```python
from build123d import *

# Parameters (mm, degrees)
F0_R     = 4.5
F1_DEPTH = 10


with BuildPart() as f1:
    # F0 (on Top) → F1 (new body)
    with BuildSketch(Plane.XY):
        with BuildLine():
            ThreePointArc((-2.392851, 5.821348), (-2.36707, 5.442285), (-2.615174, 5.154538))
            ThreePointArc((-2.615174, 5.154538), (-2.753594, 5.081941), (-2.89, 5.005627))
            ThreePointArc((-2.89, 5.005627), (-3.024293, 4.925652), (-3.156374, 4.842076))
            ThreePointArc((-3.156374, 4.842076), (-3.529622, 4.771085), (-3.84501, 4.982943))
            ThreePointArc((-3.84501, 4.982943), (-5.394961, 6.242549), (-7.385022, 6.411696))
            Line((-7.385022, 6.411696), (-7.492977, 6.287354))
            Line((-7.492977, 6.287354), (-7.596684, 6.159448))
            ThreePointArc((-7.596684, 6.159448), (-7.084536, 4.228992), (-5.57492, 2.921316))
            ThreePointArc((-5.57492, 2.921316), (-5.311514, 2.647509), (-5.316613, 2.267604))
            ThreePointArc((-5.316613, 2.267604), (-5.375984, 2.123017), (-5.431423, 1.976876))
            ThreePointArc((-5.431423, 1.976876), (-5.482891, 1.829291), (-5.53035, 1.680367))
            ThreePointArc((-5.53035, 1.680367), (-5.770641, 1.386066), (-6.148423, 1.345631))
            ThreePointArc((-6.148423, 1.345631), (-8.145413, 1.314256), (-9.778614, 0.164643))
            Line((-9.778614, 0.164643), (-9.781386, 0))
            Line((-9.781386, 0), (-9.778614, -0.164643))
            ThreePointArc((-9.778614, -0.164643), (-8.145413, -1.314256), (-6.148423, -1.345631))
            ThreePointArc((-6.148423, -1.345631), (-5.770641, -1.386066), (-5.53035, -1.680367))
            ThreePointArc((-5.53035, -1.680367), (-5.482891, -1.829291), (-5.431423, -1.976876))
            ThreePointArc((-5.431423, -1.976876), (-5.375984, -2.123017), (-5.316613, -2.267604))
            ThreePointArc((-5.316613, -2.267604), (-5.311514, -2.647509), (-5.57492, -2.921316))
            ThreePointArc((-5.57492, -2.921316), (-7.084536, -4.228992), (-7.596684, -6.159448))
            Line((-7.596684, -6.159448), (-7.492977, -6.287354))
            Line((-7.492977, -6.287354), (-7.385022, -6.411696))
            ThreePointArc((-7.385022, -6.411696), (-5.394961, -6.242549), (-3.84501, -4.982943))
            ThreePointArc((-3.84501, -4.982943), (-3.529622, -4.771085), (-3.156374, -4.842076))
            ThreePointArc((-3.156374, -4.842076), (-3.024293, -4.925652), (-2.89, -5.005627))
            ThreePointArc((-2.89, -5.005627), (-2.753594, -5.081941), (-2.615174, -5.154538))
            ThreePointArc((-2.615174, -5.154538), (-2.36707, -5.442285), (-2.392851, -5.821348))
            ThreePointArc((-2.392851, -5.821348), (-2.708726, -7.793448), (-1.860181, -9.601465))
            Line((-1.860181, -9.601465), (-1.69852, -9.632785))
            Line((-1.69852, -9.632785), (-1.535897, -9.658645))
            ThreePointArc((-1.535897, -9.658645), (-0.120147, -8.249884), (0.257526, -6.288681))
            ThreePointArc((0.257526, -6.288681), (0.362947, -5.92366), (0.694504, -5.738124))
            ThreePointArc((0.694504, -5.738124), (0.849406, -5.717247), (1.003686, -5.692189))
            ThreePointArc((1.003686, -5.692189), (1.157233, -5.662968), (1.309934, -5.629607))
            ThreePointArc((1.309934, -5.629607), (1.684953, -5.690555), (1.90886, -5.997506))
            ThreePointArc((1.90886, -5.997506), (2.934527, -7.711263), (4.746722, -8.55085))
            Line((4.746722, -8.55085), (4.890693, -8.470929))
            Line((4.890693, -8.470929), (5.031892, -8.386207))
            ThreePointArc((5.031892, -8.386207), (5.210886, -6.397007), (4.239562, -4.651875))
            ThreePointArc((4.239562, -4.651875), (4.085689, -4.304489), (4.220415, -3.94924))
            ThreePointArc((4.220415, -3.94924), (4.325658, -3.833678), (4.427737, -3.715312))
            ThreePointArc((4.427737, -3.715312), (4.526578, -3.59423), (4.622109, -3.47052))
            ThreePointArc((4.622109, -3.47052), (4.948567, -3.276151), (5.317394, -3.367364))
            ThreePointArc((5.317394, -3.367364), (7.204682, -4.020892), (9.13258, -3.499197))
            Line((9.13258, -3.499197), (9.191496, -3.345431))
            Line((9.191496, -3.345431), (9.245203, -3.189769))
            ThreePointArc((9.245203, -3.189769), (8.103686, -1.550899), (6.23786, -0.838405))
            ThreePointArc((6.23786, -0.838405), (5.896692, -0.6712), (5.771548, -0.312462))
            ThreePointArc((5.771548, -0.312462), (5.777887, -0.156288), (5.78, 0))
            ThreePointArc((5.78, 0), (5.777887, 0.156288), (5.771548, 0.312462))
            ThreePointArc((5.771548, 0.312462), (5.896692, 0.6712), (6.23786, 0.838405))
            ThreePointArc((6.23786, 0.838405), (8.103686, 1.550899), (9.245203, 3.189769))
            Line((9.245203, 3.189769), (9.191496, 3.345431))
            Line((9.191496, 3.345431), (9.13258, 3.499197))
            ThreePointArc((9.13258, 3.499197), (7.204682, 4.020892), (5.317394, 3.367364))
            ThreePointArc((5.317394, 3.367364), (4.948567, 3.276151), (4.622109, 3.47052))
            ThreePointArc((4.622109, 3.47052), (4.526578, 3.59423), (4.427737, 3.715312))
            ThreePointArc((4.427737, 3.715312), (4.325658, 3.833678), (4.220415, 3.94924))
            ThreePointArc((4.220415, 3.94924), (4.085689, 4.304489), (4.239562, 4.651875))
            ThreePointArc((4.239562, 4.651875), (5.210886, 6.397007), (5.031892, 8.386207))
            Line((5.031892, 8.386207), (4.890693, 8.470929))
            Line((4.890693, 8.470929), (4.746722, 8.55085))
            ThreePointArc((4.746722, 8.55085), (2.934527, 7.711263), (1.90886, 5.997506))
            ThreePointArc((1.90886, 5.997506), (1.684953, 5.690555), (1.309934, 5.629607))
            ThreePointArc((1.309934, 5.629607), (1.157233, 5.662968), (1.003686, 5.692189))
            ThreePointArc((1.003686, 5.692189), (0.849406, 5.717247), (0.694504, 5.738124))
            ThreePointArc((0.694504, 5.738124), (0.362947, 5.92366), (0.257526, 6.288681))
            ThreePointArc((0.257526, 6.288681), (-0.120147, 8.249884), (-1.535897, 9.658645))
            Line((-1.535897, 9.658645), (-1.69852, 9.632785))
            Line((-1.69852, 9.632785), (-1.860181, 9.601465))
            ThreePointArc((-1.860181, 9.601465), (-2.708726, 7.793448), (-2.392851, 5.821348))
        make_face()
        Circle(F0_R, mode=Mode.SUBTRACT)
    extrude(amount=F1_DEPTH)


solid = f1.part
```
Geometry: final body of the model. Coordinates: model frame, mm. A direction names the side the tool comes from. Coordinates: 2 decimals unless noted, no trailing zeros. Write each loop counter-clockwise with the first axis right and the second up, starting at its lowest first coordinate (ties: lowest second). Pieces come first, ordered by that corner, then holes. Notation, with made-up numbers: M -20.75,-2.5 L 28.25,-2.5 A29 ccw 28.25,26.5 Z; hole C 24,59.25 d3. An arc over 180 degrees is marked long. Use CSV: the item, a comma, the result in double quotes. Start each with the question number.
1. Reachability of faces 1 (the face through (-8.172, -1.305, 4.93)), 2 (the face through (-7.099, 4.253, 4.93)), 3 (the face through (8.13, -1.57, 4.93)) from +Z, -Z, +X, -X, +Y, -Y: full face, straight path, thin tool, end or side. Return the list, or none.
2. First-contact query: P1, Ø2, axis at y = -4.5, z = 1, coming from the -X side; P2, Ø3, axis at y = 3.5, z = 7, coming from the -X side; P3, Ø4, axis at x = 2, z = 3.5, coming from the -Y side. Flat tips, straight axial feed; report the tip coordinate or a pass-through.
3. Cut plane B-B on y = 7.75. Return the cut outline in (x, z).
4. Ray query, probe 1 along Y at (x, z) = (-6.5, 6); probe 2 along Y at (x, z) = (0, 7.25); probe 3 along Y at (x, z) = (-1, 9). Return the intervals inside material, ascending.
5. Mould query, pull axis Y, two halves, no side actions, for faces 4 (the face through (-5, 1, 0)), 5 (the face through (-0.59, 4.46, 4.93)), 6 (the face through (7.18, -4.02, 4.93)). Classes: pulls with the +Y half, pulls with the -Y half, needs draft (parallel to the pull), parting line crosses it, or undercut.
6. Cut plane A-A on x = 0. Return the cut outline in (y, z).
Entries:
1,face 1,"+Z, -Z"
1,face 2,"+Z, -Z, -X"
1,face 3,"+Z, -Z, +X"
2,P1,"x = -7.56"
2,P2,"x = -7.44"
2,P3,"y = -8.36"
3,outline,"M -2.71,0 L 0.1,0 L 0.1,10 L -2.71,10 Z; M 2.98,0 L 5.22,0 L 5.22,10 L 2.98,10 Z"
4,probe 1,"-6.49 to -3.53, -1.43 to 1.43, 3.53 to 6.49"
4,probe 2,"-8 to -4.5, 4.5 to 8"
4,probe 3,"-9.31 to -4.39, 4.39 to 9.31"
5,face 4,"needs draft"
5,face 5,"undercut"
5,face 6,"pulls with the -Y half"
6,outline,"M -8,0 L -4.5,0 L -4.5,10 L -8,10 Z; M 4.5,0 L 8,0 L 8,10 L 4.5,10 Z"
